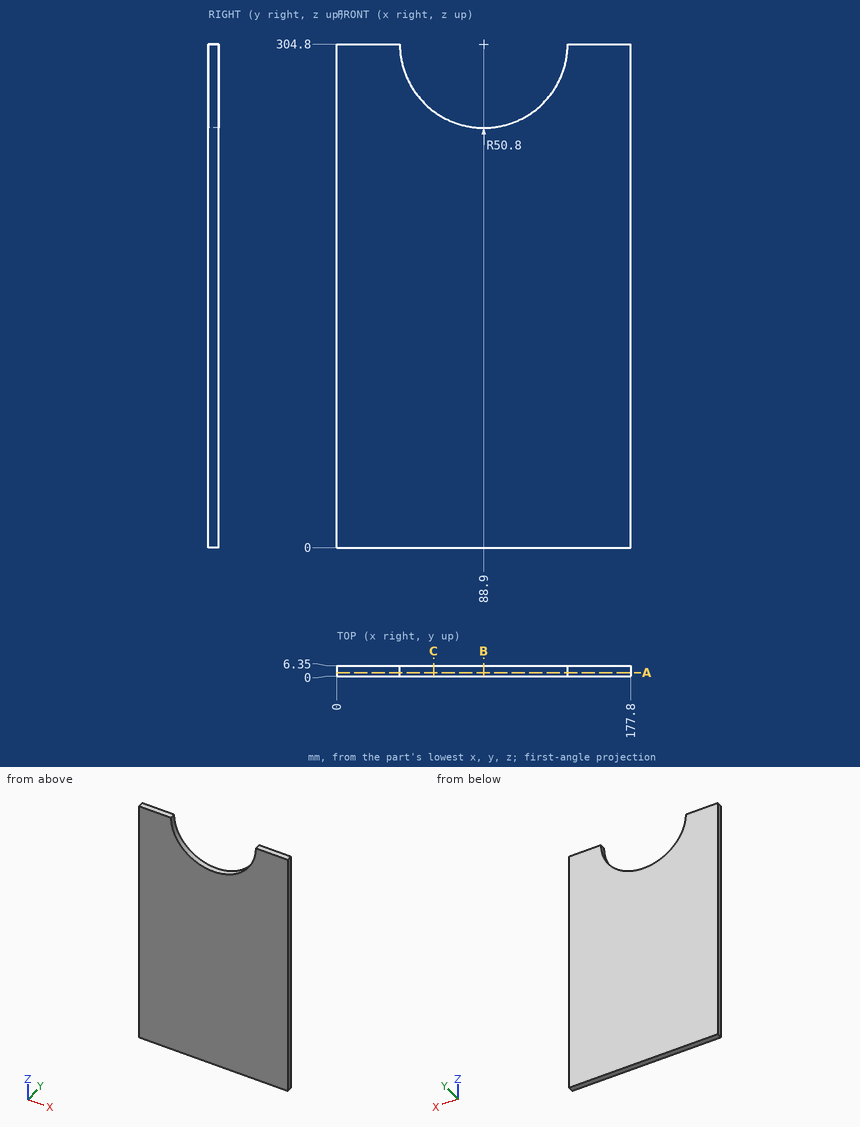
The drawing under review shows one solid part. Ordinate dimensions are in mm from its lowest x, y, z. Round coordinates to 2 decimals unless told otherwise and drop trailing zeros. Write each loop counter-clockwise with the first axis right and the second up, starting at its lowest first coordinate (ties: lowest second). Pieces come first, ordered by that corner, then holes.
(1) We need section B-B on x = 88.9. Give the boundary of the cut face in (y, z).
(2) Wall thickness on L1, parallel to X at y = 3.25, z = 263; L2, parallel to Z at x = 133, y = 6.25; L3, parallel to Z at x = 108, y = 4.5: over which ranges is each line inside the solid? List them lowest first.
(3) We need section C-C on x = 58.5. Give the boundary of the cut face in (y, z), and give its area (3 significant figures).
(4) We need section A-A on y = 2. Give the boundary of the cut face in (x, z), and give its area (3 significant figures).
Findings below:
1. outline: (0, 0) - (6.35, 0) - (6.35, 254) - (0, 254) - close
2. L1: x = 0 to 60.03, 117.77 to 177.8
2. L2: z = 0 to 279.58
2. L3: z = 0 to 257.73
3. outline: (0, 0) - (6.35, 0) - (6.35, 264.1) - (0, 264.1) - close
3. area: 1,680 mm2
4. outline: (0, 0) - (177.8, 0) - (177.8, 304.8) - (139.7, 304.8) arc R50.8 cw to (38.1, 304.8) - (0, 304.8) - close
4. area: 50,100 mm2
